Model file for the job. Use its own axes, mm. A direction names the side the tool comes from. Coordinates: 2 decimals unless noted, no trailing zeros. Order: outer loops, then holes, each group sorted by start corner. A loop starts at its lowest first (then second) coordinate and runs counter-clockwise, first axis right, second up. Notation, with made-up numbers: (56, -26) -> (91, -26) arc R14 ccw to (91, -18) -> close; hole circle Ø9 at (0.25, -24.75). An arc over 180 degrees is marked (long way). Write item = value, one per line. Start each with the question number.
Q1. Cut at C-C, the plane x = -98. List the corners of the cut face in (y, z), plus the area to 3 significant figures.
Q2. Cut at B-B, the plane z = 33. List the corners of the cut face in (x, y), plus the area to 3 significant figures.
Q3. Cut at D-D, the plane x = -165. List the corners of the cut face in (y, z).
Q4. Mould opens along Y. For faces 1 (the face through (-74.005, -46.133, 59.203)), 2 (the face through (-51.813, -19.15, 59.203)), 3 (the face through (-196, -27, 43)) say: +Y half, -Y half, draft (parallel to the pull), parting line (faces both ways), or undercut.
Q5. Wall check: line 1 (Y direction, x = -41, z = 0); line 2 (X direction, y = -18, z = 60); line 3 (Y direction, x = -95, z = 59.5). Give the ranges that are in metal, low to high. Write a range as from..to.
Q6. Flat gauge pins, fed straight in: pin 1 (4 mm diameter, centred on x = -153, z = 38.5, fed in from -Y); pin 2 (10 mm diameter, centred on y = 27, z = 82.5, fed in from +X); pin 3 (3 mm diameter, centred on y = 22, z = 59.5, fed in from +X). Where does each tip first touch, or does it go through?
Q7. Cut at A-A, the plane y = 0. List the corners of the cut face in (x, z).
Q8. 3-axis set-ups, long thin cutter, end or side, ignore diameter. For faces 4 (the face through (-96.628, -11.273, -50.763)), 5 (the face through (-96.63, 23.07, -44.36)): which of +Z, -Z, +X, -X, +Y, -Y reach the whole face in a straight line?
from build123d import *

# Parameters (mm, degrees)
F0_R     = 52
F0_R_2   = 50
F2_DEPTH = 196
F1_R     = 52
F1_R_2   = 50
F3_DEPTH = 98
F4_DEPTH = 78
F5_DEPTH = 188


with BuildPart() as f2:
    # F0 (on Right) → F2 (new body)
    with BuildSketch(Plane.YZ):
        Circle(F0_R)
        Circle(F0_R_2, mode=Mode.SUBTRACT)
    extrude(amount=-F2_DEPTH)

    # F1 (on Top) → F3 (join)
    with BuildSketch(Plane.XY):
        with Locations((-98, 0)):
            Circle(F1_R)
        with Locations((-98, 0)):
            Circle(F1_R_2, mode=Mode.SUBTRACT)
    extrude(amount=F3_DEPTH)

    # F1 (on Top) → F4 (cut)
    with BuildSketch(Plane.XY):
        with Locations((-98, 0)):
            Circle(F1_R_2)
    extrude(amount=F4_DEPTH, mode=Mode.SUBTRACT)

    # F0 (on Right) → F5 (cut)
    with BuildSketch(Plane.YZ):
        Circle(F0_R_2)
    extrude(amount=-F5_DEPTH, mode=Mode.SUBTRACT)


solid = f2.part
Here are the results:
q1.outline = (-52, 0) arc R52 ccw to (52, 0) -> (52, 98) -> (50, 98) -> (50, 0) arc R50 cw to (-50, 0) -> (-50, 98) -> (-52, 98) -> close
q1.area = 712 mm²
q2.outline = (-196, -40.19) -> (-131, -40.19) arc R52 ccw to (-65, -40.19) -> (0, -40.19) -> (0, -37.56) -> (-65, -37.56) arc R50 cw to (-131, -37.56) -> (-196, -37.56) -> close; (-196, 37.56) -> (-131, 37.56) arc R50 cw to (-65, 37.56) -> (0, 37.56) -> (0, 40.19) -> (-65, 40.19) arc R52 ccw to (-131, 40.19) -> (-196, 40.19) -> close
q2.area = 969 mm²
q3.outline = circle Ø104 at (0, 0); hole circle Ø100 at (0, 0)
q4.face_1 = parting line
q4.face_2 = undercut
q4.face_3 = draft
q5.line_1 = -52..-50, 50..52
q5.line_2 = -146.79..-144.65, -51.35..-49.21
q5.line_3 = -51.91..-49.91, 49.91..51.91
q6.pin_1 = -37.04
q6.pin_2 = -50.88
q6.pin_3 = -50.21
q7.outline = (-196, -52) -> (0, -52) -> (0, -50) -> (-196, -50) -> close; (-196, 50) -> (-148, 50) -> (-148, 98) -> (-150, 98) -> (-150, 52) -> (-196, 52) -> close; (-48, 50) -> (0, 50) -> (0, 52) -> (-46, 52) -> (-46, 98) -> (-48, 98) -> close
q8.face_4 = none
q8.face_5 = +X, -X
